Geometry: final body of the model. Coordinates: model frame, mm. A direction names the side the tool comes from. Round coordinates to 2 decimals unless told otherwise and drop trailing zeros. Loops run counter-clockwise (first coordinate to the right, second up) from the corner with the lowest first, then second, coordinate; pieces in that order, holes last. Notation, with made-up numbers: (20.5, -12) - (53.5, -12) arc R26 cw to (53.5, 12) - close; hole circle Ø2 at (23, 39). An arc over 180 degrees is marked (long way). Answer as a JSON object with one key per item and string values. Group by question number.
Item 1: Draft query along X for faces 5 (the face through (-82.81, 9.88, -130.65)), 6 (the face through (-7.2, 10.5, -130.6)), 7 (the face through (0, 7.285, -131)). Return one class per face: released by +X, released by -X, zero draft, split by the parting line, or undercut.
Item 2: Section A-A (x = -100). Return the cut outline in (y, z) (3 decimals), plus the area to 3 significant figures.
Item 3: Reachability of faces 1 (the face through (13, 19.35, -131)), 2 (the face through (-19.35, -12, -131)), 3 (the face through (-7.285, 0, -131)), 4 (the face through (-10, 19.35, -131)) from +Z, -Z, +X, -X, +Y, -Y: full face, straight path, thin tool, end or side. Return the list, or none.
Item 4: First-contact query: pin 1 (4 mm diameter, centred on y = 18, z = -178, fed in from +X); pin 2 (3 mm diameter, centred on y = -0.5, z = -174.5, fed in from +X) (3 decimals); pin 3 (1.5 mm diameter, centred on x = -71, z = -107, fed in from +Y); pin 4 (3 mm diameter, centred on x = -100.5, z = -118.5, fed in from +Y). Flat tips, straight axial feed; report the tip coordinate or a pass-through.
Item 5: Line query: line 1 (Y direction, x = -104, z = -10); line 2 (X direction, y = 12, z = -59.5); line 3 (X direction, y = 12.5, z = -115.5). Output: solid intervals per line, ascending.
```python
from build123d import *

# Parameters (mm, degrees)
BOSS_EXTRUDE1_DEPTH = 265
SKETCH3_R           = 1.65
CUT_EXTRUDE1_DEPTH  = 40


with BuildPart() as part:
    # Sketch2 → Boss-Extrude1 (new body)
    with BuildSketch(Plane.XY):
        with BuildLine():
            ThreePointArc((-3.764, 17.3228), (-4.357753133, 18.756246867), (-5.7912, 19.35))
            Line((-5.7912, 19.35), (-6.964305235, 19.35))
            Line((-6.964305235, 19.35), (-8.996305235, 19.35))
            Line((-8.996305235, 19.35), (-13.723477062, 19.35))
            Line((-13.723477062, 19.35), (-15.821601592, 19.115365338))
            ThreePointArc((-15.821601592, 19.115365338), (-17.870947824, 17.870947824), (-19.115365338, 15.821601592))
            Line((-19.115365338, 15.821601592), (-19.35, 6.964305235))
            Line((-19.35, 6.964305235), (-19.35, 5.7912))
            ThreePointArc((-19.35, 5.7912), (-18.756246867, 4.357753133), (-17.3228, 3.764))
            Line((-17.3228, 3.764), (-16.7132, 3.764))
            ThreePointArc((-16.7132, 3.764), (-15.279753133, 4.357753133), (-14.686, 5.7912))
            Line((-14.686, 5.7912), (-14.686, 8.996305235))
            ThreePointArc((-14.686, 8.996305235), (-14.074427708, 9.911587851), (-12.994778249, 9.696832221))
            Line((-12.994778249, 9.696832221), (-8.101029797, 4.803083769))
            ThreePointArc((-8.101029797, 4.803083769), (-7.497079234, 3.899207877), (-7.285, 2.833013566))
            Line((-7.285, 2.833013566), (-7.285, -2.833013566))
            ThreePointArc((-7.285, -2.833013566), (-7.497079234, -3.899207877), (-8.101029797, -4.803083769))
            Line((-8.101029797, -4.803083769), (-12.994778249, -9.696832221))
            ThreePointArc((-12.994778249, -9.696832221), (-14.074427708, -9.911587851), (-14.686, -8.996305235))
            Line((-14.686, -8.996305235), (-14.686, -5.7912))
            ThreePointArc((-14.686, -5.7912), (-15.279753133, -4.357753133), (-16.7132, -3.764))
            Line((-16.7132, -3.764), (-17.3228, -3.764))
            ThreePointArc((-17.3228, -3.764), (-18.756246867, -4.357753133), (-19.35, -5.7912))
            Line((-19.35, -5.7912), (-19.35, -6.964305235))
            Line((-19.35, -6.964305235), (-19.35, -19.05))
            Line((-19.35, -19.05), (-118.649495781, -19.05))
            Line((-118.649495781, -19.05), (-118.649495781, -9.05))
            Line((-118.649495781, -9.05), (-45.95, 29.35))
            Line((-45.95, 29.35), (19.05, 29.35))
            Line((19.05, 29.35), (19.05, 19.35))
            Line((19.05, 19.35), (6.964305235, 19.35))
            Line((6.964305235, 19.35), (5.7912, 19.35))
            ThreePointArc((5.7912, 19.35), (4.357753133, 18.756246867), (3.764, 17.3228))
            Line((3.764, 17.3228), (3.764, 16.7132))
            ThreePointArc((3.764, 16.7132), (4.357753133, 15.279753133), (5.7912, 14.686))
            Line((5.7912, 14.686), (8.996305235, 14.686))
            ThreePointArc((8.996305235, 14.686), (9.911587851, 14.074427708), (9.696832221, 12.994778249))
            Line((9.696832221, 12.994778249), (4.803083769, 8.101029797))
            ThreePointArc((4.803083769, 8.101029797), (3.899207877, 7.497079234), (2.833013566, 7.285))
            Line((2.833013566, 7.285), (-2.833013566, 7.285))
            ThreePointArc((-2.833013566, 7.285), (-3.899207877, 7.497079234), (-4.803083769, 8.101029797))
            Line((-4.803083769, 8.101029797), (-9.696832221, 12.994778249))
            ThreePointArc((-9.696832221, 12.994778249), (-9.911587851, 14.074427708), (-8.996305235, 14.686))
            Line((-8.996305235, 14.686), (-5.7912, 14.686))
            ThreePointArc((-5.7912, 14.686), (-4.357753133, 15.279753133), (-3.764, 16.7132))
            Line((-3.764, 16.7132), (-3.764, 17.3228))
        make_face()
    extrude(amount=-BOSS_EXTRUDE1_DEPTH)

    # Sketch3 → Cut-Extrude1 (cut)
    with BuildSketch(Plane.ZY.offset(118.649495781)):
        with Locations((-10, -14.05)):
            Circle(SKETCH3_R)
        with Locations((-275.03, -14.05)):
            Circle(SKETCH3_R)
        with Locations((-142.515, -14.05)):
            Circle(SKETCH3_R)
    extrude(amount=-CUT_EXTRUDE1_DEPTH, mode=Mode.SUBTRACT)


solid = part.part
```
Values:
{
 "1": {"face 5": "released by -X", "face 6": "undercut", "face 7": "zero draft"},
 "2": {"outline": "(-19.05, -265) - (0.801, -265) - (0.801, 0) - (-19.05, 0) - close; hole circle Ø3.3 at (-14.05, -142.515); hole circle Ø3.3 at (-14.05, -10)", "area": "5,240 mm^2"},
 "3": {"face 1": "+Z, -Z, +X", "face 2": "+Z, -Z, -Y", "face 3": "+Z, -Z, +X, -Y", "face 4": "+Z, -Z"},
 "4": {"pin 1": "stops at x = 19.05", "pin 2": "stops at x = -7.285", "pin 3": "stops at y = 16.51", "pin 4": "stops at y = 1.33"},
 "5": {"line 1": "y = -19.05 to -15.7, -12.4 to -1.31", "line 2": "x = -78.8 to -19.22, -8.7 to 8.7", "line 3": "x = -77.85 to -19.2, -9.2 to 9.2"}
}
